```python
from build123d import *

# Parameters (mm, degrees)
EXTRUDE_1_DEPTH     = 10
FILLET_1_R          = 55.243368
FILLET_2_R          = 90.446111
CUT_EXTRUDE_1_DEPTH = 10


with BuildPart() as part:
    # 草图1 → 凸台-拉伸1 (new body)
    with BuildSketch(Plane.XY):
        Polygon((424.616260913, 129.386586507), (424.616260913, -70.613413493), (-74.025647104, -33.786146841), (-74.025647104, 66.213853159), align=None)
    extrude(amount=EXTRUDE_1_DEPTH)

    # 圆角1
    fillet_1_edges = [part.edges().sort_by_distance(p)[0] for p in [
        (-74.025647104, -33.786146841, 5),
        (-74.025647104, 66.213853159, 5),
    ]]
    fillet(fillet_1_edges, radius=FILLET_1_R - 0.0001)  # a hair under: the kernel refuses the full size

    # 圆角2
    fillet_2_edges = [part.edges().sort_by_distance(p)[0] for p in [
        (424.616260913, 129.386586507, 5),
        (424.616260913, -70.613413493, 5),
    ]]
    fillet(fillet_2_edges, radius=FILLET_2_R - 0.0001)  # a hair under: the kernel refuses the full size

    # 草图2 → 切除-拉伸1 (cut)
    with BuildSketch(Plane.XY.offset(10)):
        with BuildLine():
            Line((-28.487167505, 58.083637567), (333.136967432, 103.286654435))
            ThreePointArc((333.136967432, 103.286654435), (408.475328877, 27.948292989), (333.136967432, -47.390068456))
            Line((333.136967432, -47.390068456), (-18.353743943, -22.983750924))
            ThreePointArc((-18.353743943, -22.983750924), (-63.95414997, 12.483231541), (-28.487167505, 58.083637567))
        make_face()
    extrude(amount=-CUT_EXTRUDE_1_DEPTH, mode=Mode.SUBTRACT)


solid = part.part
```
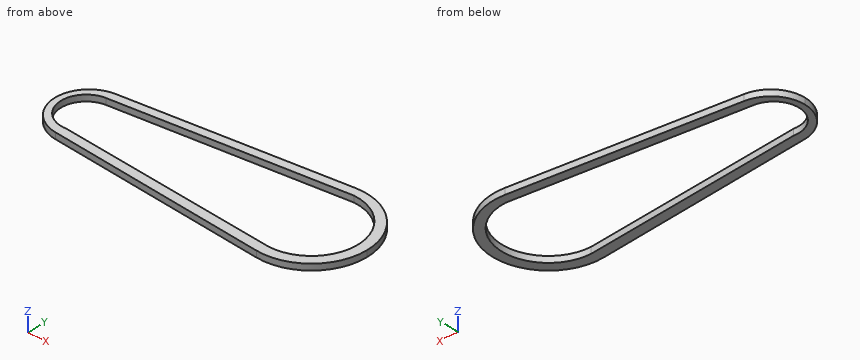
CAD build for the part. Positions are in the model's coordinates, mm. Coordinates: 2 decimals unless noted, no trailing zeros. Order: outer loops, then holes, each group sorted by start corner. A loop starts at its lowest first (then second) coordinate and runs counter-clockwise, first axis right, second up. Notation, with made-up numbers: (-32, -33) -> (-18, -33) arc R23 cw to (-18, -5) -> close; hole circle Ø5 at (-29.5, 2). An arc over 180 degrees is marked (long way). Use one line per item in the form item = value. Start each with the question number.
1) Drop flat-ended pins along their axis: pin 1 (4 mm diameter, centred on x = 233, z = 6, fed in from +Y); pin 2 (5 mm diameter, centred on y = -23.5, z = 5, fed in from +X); pin 3 (1 mm diameter, centred on x = 367, z = 4.5, fed in from +Y). Give the stop position or say it passes through.
2) Drill centre lines: L1, parallel to Y at x = 96.5, z = 7; L2, parallel to Y at x = 260, z = 3.5; L3, parallel to X at y = 35.5, z = 2.5. Where is each one in solid material? Low to high. Write a range as [from, to].
3) Band-saw the part on A-A on x = 105. Give the cut face in (y, z), then the cut area to 3 significant figures.
4) Band-saw the part on B-B on y = -17.5. Give the cut face in (x, z).
Entries:
q1.pin_1 = 105.36
q1.pin_2 = 410.98
q1.pin_3 = 111.23
q2.L1 = [-46.38, -30.96], [73.71, 87.82]
q2.L2 = [-58.46, -42.31], [94.14, 108.53]
q2.L3 = [-71.02, -60.11], [408.1, 424.19]
q3.outline = (-47.01, 0) -> (-31.55, 0) -> (-31.55, 10) -> (-47.01, 10) -> close; (74.77, 0) -> (88.89, 0) -> (88.89, 10) -> (74.77, 10) -> close
q3.area = 296 mm2
q4.outline = (-61.5, 0) -> (-44.4, 0) -> (-44.4, 10) -> (-61.5, 10) -> close; (393.22, 0) -> (413.05, 0) -> (413.05, 10) -> (393.22, 10) -> close
